Solid Edge part; units mm, degrees
sketch "Sketch1" plane through (0, 0, 0) normal (0, 0, 1) x (1, 0, 0)
  line L0 (0, 30) -> (0, 27.575)
  line L1 (0, 27.575) -> (4.6268, 27.575)
  arc A0 (4.6268, 27.575) -> (10.1272, 25.2875) centre (5.95, 23) cw
  line L2 (10.1272, 25.2875) -> (13.6728, 25.2875)
  arc A1 (13.6728, 25.2875) -> (19.1732, 27.575) centre (17.85, 23) cw
  line L3 (19.1732, 27.575) -> (23.8, 27.575)
  line L4 (23.8, 27.575) -> (23.8, 30)
  arc A2 (23.8, 30) -> (22.8, 31) centre (22.8, 30) ccw
  line L5 (22.8, 31) -> (1, 31)
  arc A3 (1, 31) -> (0, 30) centre (1, 30) ccw
revolve "RevolvedProtrusion1" add sketch "Sketch1" angle 360 about axis through (23.8, 0, 0) along (-1, 0, 0)
properties part number "3206 A-2RS1_PART2"
Check sheet for the modelled part. Datum: model origin and axes. Units: mm. Give positions to 0.01 mm unless a question says otherwise; leave off trailing zeros. Loops run counter-clockwise (first coordinate to the right, second up) from the corner with the lowest first, then second, coordinate; pieces in that order, holes last. Notation, with made-up numbers: M 39,-23.5 L 58,-23.5 A12 cw 58,-15.5 Z; hole C -37.75,39 d6. An arc over 180 degrees is marked long. Return JSON: item names as keys, results as strings. Group by question number.
1. Cross-section at D-D on x = 14.75. Record the boundary of the cut face in (y, z).
2. Cross-section at C-C on x = 6.5. Record the boundary of the cut face in (y, z).
3. Go/stop test with flat-tipped pins: pin 1 (2 mm diameter, centred on x = 9, y = -19, fed in from +Z); pin 2 (4 mm diameter, centred on x = 12.5, y = 4.5, fed in from +Z); pin 3 (12 mm diameter, centred on x = 15, z = 22.5, fed in from +Y); pin 4 (2 mm diameter, centred on y = 12, z = -24.5, fed in from +X). Record where each tip stops, or that it passes through.
4. Thickness scan on L1, parallel to Y at x = 20.55, z = 0 (3 decimals); L2, parallel to Y at x = 11.2, z = 0. Record the ranges inside material, lowest first.
5. Mould release check, pull along Y, two halves, no side actions. Record for faces 1 (the cylindrical face through (21.519, 25.472, -10.561)), 2 (the flat face through (23.8, 9, 27)), 3 (the cylindrical face through (2.35, -21.88, -16.78)), 4 (the cylindrical face through (11.747, -4.036, -30.736)): released by +Y, released by -Y, zero draft, split by the parting line, or undercut.
Return value:
{
 "1": {"outline": "C 0,0 d62; hole C 0,0 d53.23"},
 "2": {"outline": "C 0,0 d62; hole C 0,0 d55.46"},
 "3": {"pin 1": "z = 25.24", "pin 2": "z = 30.9", "pin 3": "y = 26.24", "pin 4": "x = 23.8"},
 "4": {"L1": "-31 to -27.575, 27.575 to 31", "L2": "-31 to -25.29, 25.29 to 31"},
 "5": {"face 1": "undercut", "face 2": "zero draft", "face 3": "undercut", "face 4": "split by the parting line"}
}
